Design review of the part shown in the three views and the two pictorial views. Dimensions are in mm from the part's minimum x, y and z. A direction names the side the tool comes from. Round coordinates to 2 decimals unless told otherwise and drop trailing zeros. Order: outer loops, then holes, each group sorted by start corner. A loop starts at its lowest first (then second) coordinate and runs counter-clockwise, first axis right, second up. Notation, with made-up numbers: (-18.5, -18.75) - (27.5, -18.75) arc R8 ccw to (27.5, -5.75) - close; hole circle Ø8 at (56, -17). An arc over 180 degrees is marked (long way). Use CSV: the item, a comma, the result in double quotes.
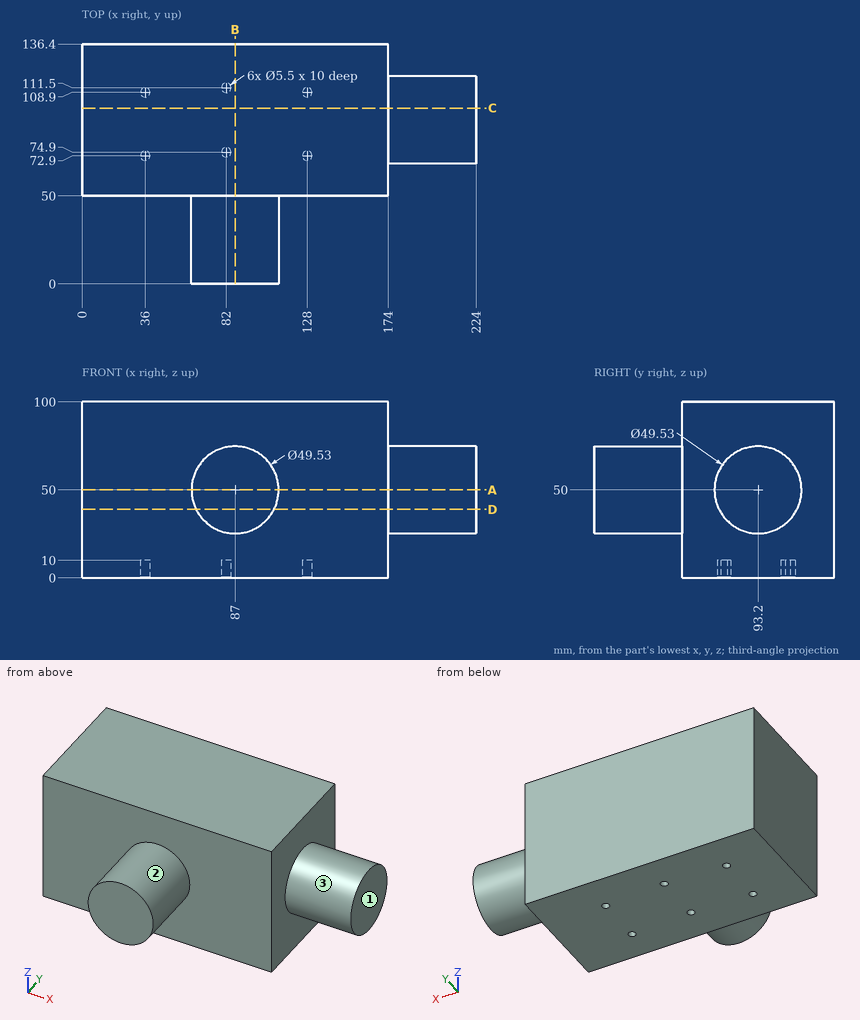
1) We need section D-D (z = 39). Give the boundary of the cut face in (x, y), then the cut area to 3 significant figures.
Data:
outline,"(0, 50) - (64.81, 50) - (64.81, 0) - (109.19, 0) - (109.19, 50) - (174, 50) - (174, 71.01) - (224, 71.01) - (224, 115.39) - (174, 115.39) - (174, 136.4) - (0, 136.4) - close"
area,"19,500 mm2"
2) Insertion check: pin 1 Ø1.5 at (x, y) = (150.5, 122.5) entering from -Z; pin 2 Ø1.6 at (x, y) = (82.5, 75) entering from -Z. Each pin has a flat end and moves straight along its axis. Give the tip position at first contact, or say it passes through.
Data:
pin 1,"stops at z = 0"
pin 2,"stops at z = 10"
3) To check wall thickness, follow L1, parallel to Y at x = 128, z = 4; L2, parallel to X at y = 118, z = 92.5; L3, parallel to X at y = 72, z = 3. State the ranges of each line that lie inside material, in increasing order. Write a range as from..to.
Data:
L1,"y = 50..70.15, 75.65..106.15, 111.65..136.4"
L2,"x = 0..174"
L3,"x = 0..33.4, 38.6..125.4, 130.6..174"
4) We need section C-C (y = 100). Give the boundary of the cut face in (x, z), then the cut area to 3 significant figures.
Data:
outline,"(0, 0) - (174, 0) - (174, 26.19) - (224, 26.19) - (224, 73.81) - (174, 73.81) - (174, 100) - (0, 100) - close"
area,"19,800 mm2"
5) For the marked faces 1, 2 and 3, list the 3-axis set-ups (+Z, -Z, +X, -X, +Y, -Y) from which the entire face can be reached by the end or side of a thin tool; tool diameter is ignored.
Data:
face 1,"+Z, -Z, +X, +Y, -Y"
face 2,"-Y"
face 3,"+X"
6) We need section A-A (z = 50). Give the boundary of the cut face in (x, y) (3 decimals), then the cut area to 3 significant figures.
Data:
outline,"(0, 50) - (62.235, 50) - (62.235, 0) - (111.765, 0) - (111.765, 50) - (174, 50) - (174, 68.435) - (224, 68.435) - (224, 117.965) - (174, 117.965) - (174, 136.4) - (0, 136.4) - close"
area,"20,000 mm2"
7) We need section B-B (x = 87). Give the boundary of the cut face in (y, z) (3 decimals).
Data:
outline,"(0, 25.235) - (50, 25.235) - (50, 0) - (136.4, 0) - (136.4, 100) - (50, 100) - (50, 74.765) - (0, 74.765) - close"
